Part model, mm, in its own coordinate system. Face numbers are marked on the shaded views. A direction names the side the tool comes from. Coordinates: 2 decimals unless noted, no trailing zeros. Write each loop counter-clockwise with the first axis right and the second up, starting at its lowest first coordinate (ties: lowest second). Pieces come first, ordered by that corner, then holes. Notation, with made-up numbers: (71.5, -33) -> (123.5, -33) arc R29 cw to (123.5, 1) -> close; hole circle Ø5 at (-6, 11.5). An arc over 180 degrees is marked (long way). Write item = value, one per line.
from build123d import *

# Parameters (mm, degrees)
BASE_FLANGE1_DEPTH = 50
EDGE_FLANGE1_DEPTH = 62
SKETCH9_W          = 25
SKETCH9_H          = 20
CUT_EXTRUDE1_DEPTH = 10
EDGE_FLANGE2_DEPTH = 21
SKETCH13_R         = 3.5
CUT_EXTRUDE2_DEPTH = 10
EDGE_FLANGE3_DEPTH = 24
SKETCH17_R         = 6.5
CUT_EXTRUDE3_DEPTH = 10


# Sheet-metal steps are written as plain solids
with BuildPart() as part:
    # Sketch1 → Base-Flange1 (new body)
    with BuildSketch(Plane.YZ):
        with BuildLine():
            Line((-52, 46), (-46, 46))
            ThreePointArc((-46, 46), (-43.171572875, 44.828427125), (-42, 42))
            Line((-42, 42), (-42, 2))
            ThreePointArc((-42, 2), (-41.414213562, 0.585786438), (-40, 0))
            Line((-40, 0), (40, 0))
            ThreePointArc((40, 0), (41.414213562, 0.585786438), (42, 2))
            Line((42, 2), (42, 42))
            ThreePointArc((42, 42), (43.171572875, 44.828427125), (46, 46))
            Line((46, 46), (52, 46))
            Line((52, 46), (52, 44))
            Line((52, 44), (46, 44))
            ThreePointArc((46, 44), (44.585786438, 43.414213562), (44, 42))
            Line((44, 42), (44, 2))
            ThreePointArc((44, 2), (42.828427125, -0.828427125), (40, -2))
            Line((40, -2), (-40, -2))
            ThreePointArc((-40, -2), (-42.828427125, -0.828427125), (-44, 2))
            Line((-44, 2), (-44, 42))
            ThreePointArc((-44, 42), (-44.585786438, 43.414213562), (-46, 44))
            Line((-46, 44), (-52, 44))
            Line((-52, 44), (-52, 46))
        make_face()
    extrude(amount=-BASE_FLANGE1_DEPTH)

    # Edge-Flange1 section (across the edge) → Edge-Flange1 (add)
    with BuildSketch(Plane(origin=(2, -31, 0), x_dir=(-1, 0, 0), z_dir=(0, 1, 0))):
        with BuildLine():
            Line((-2, 2), (-2, 40))
            Line((-2, 40), (0, 40))
            Line((0, 40), (0, 2))
            ThreePointArc((0, 2), (0.585786438, 0.585786438), (2, 0))
            Line((2, 0), (2, -2))
            ThreePointArc((2, -2), (-0.828427125, -0.828427125), (-2, 2))
        make_face()
    extrude(amount=EDGE_FLANGE1_DEPTH)

    # Sketch9 → Cut-Extrude1 (cut)
    with BuildSketch(Plane.YZ.offset(4)):
        with Locations((-14.5, 24)):
            Rectangle(SKETCH9_W, SKETCH9_H)
    extrude(amount=-CUT_EXTRUDE1_DEPTH, mode=Mode.SUBTRACT)

    # Edge-Flange2 section (across the edge) → Edge-Flange2 (add)
    with BuildSketch(Plane(origin=(4, -4, 16), x_dir=(0, 0, -1), z_dir=(0, -1, 0))):
        with BuildLine():
            Line((-2, 2), (-2, 18))
            Line((-2, 18), (0, 18))
            Line((0, 18), (0, 2))
            ThreePointArc((0, 2), (0.585786438, 0.585786438), (2, 0))
            Line((2, 0), (2, -2))
            ThreePointArc((2, -2), (-0.828427125, -0.828427125), (-2, 2))
        make_face()
    extrude(amount=EDGE_FLANGE2_DEPTH)

    # Sketch13 → Cut-Extrude2 (cut)
    with BuildSketch(Plane.XY.offset(18)):
        with Locations((17, -14.5)):
            Circle(SKETCH13_R)
    extrude(amount=-CUT_EXTRUDE2_DEPTH, mode=Mode.SUBTRACT)

    # Edge-Flange3 section (across the edge) → Edge-Flange3 (add)
    with BuildSketch(Plane(origin=(2, 7, 42), x_dir=(0, 0, -1), z_dir=(0, 1, 0))):
        with BuildLine():
            Line((-2, 2), (-2, 33))
            Line((-2, 33), (0, 33))
            Line((0, 33), (0, 2))
            ThreePointArc((0, 2), (0.585786438, 0.585786438), (2, 0))
            Line((2, 0), (2, -2))
            ThreePointArc((2, -2), (-0.828427125, -0.828427125), (-2, 2))
        make_face()
    extrude(amount=EDGE_FLANGE3_DEPTH)

    # Sketch17 → Cut-Extrude3 (cut)
    with BuildSketch(Plane.XY.offset(44)):
        with Locations((-17, 19)):
            Circle(SKETCH17_R)
    extrude(amount=-CUT_EXTRUDE3_DEPTH, mode=Mode.SUBTRACT)


solid = part.part
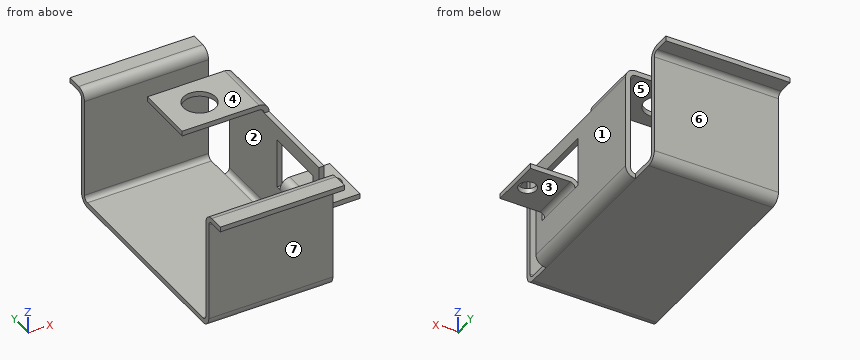
Q1. Pin check, flat tips, straight feed: pin 1 (4 mm diameter, centred on x = -40.5, y = 8, fed in from +Z); pin 2 (10 mm diameter, centred on x = 11.5, y = -15.5, fed in from -Z); pin 3 (21 mm diameter, centred on x = -17, y = 19, fed in from +Z). Stop position of each tip, or through.
Model answer:
pin_1 = 0
pin_2 = 16
pin_3 = 44
Q2. Saw through at A-A on z = 28. Give the cut face in (x, y), and give its area (3 significant figures).
Model answer:
outline = (-50, -44) -> (0, -44) -> (0, -42) -> (-50, -42) -> close; (-50, 42) -> (0, 42) -> (0, 44) -> (-50, 44) -> close; (2, -31) -> (4, -31) -> (4, -27) -> (2, -27) -> close; (2, -2) -> (4, -2) -> (4, 31) -> (2, 31) -> close
area = 274 mm²
Q3. Mould opens along Z. For the marked faces 1, 2 and 3 say: released by +Z, released by -Z, zero draft, split by the parting line, or undercut.
Model answer:
face_1 = zero draft
face_2 = undercut
face_3 = released by -Z
Q4. Saw through at C-C on z = 36.5. Give the cut face in (x, y), and give its area (3 significant figures).
Model answer:
outline = (-50, -44) -> (0, -44) -> (0, -42) -> (-50, -42) -> close; (-50, 42) -> (0, 42) -> (0, 44) -> (-50, 44) -> close; (2, -31) -> (4, -31) -> (4, 31) -> (2, 31) -> close
area = 324 mm²
Q5. Which spindle directions (+Z, -Z, +X, -X, +Y, -Y) get a long thin tool onto all of the face, cutting with end or side? Do the marked faces 4, 5, 6 and 7. Say none if no direction does.
Model answer:
face_4 = +Z, +X, -X
face_5 = -X
face_6 = -Z, +X, -X, +Y
face_7 = -Z, +X, -X, -Y
Q6. Saw through at B-B on y = -14.5. Give the cut face in (x, z), and give its area (3 significant figures).
Model answer:
outline = (-50, -2) -> (0, -2) arc R4 ccw to (4, 2) -> (4, 14) arc R2 cw to (6, 16) -> (13.5, 16) -> (13.5, 18) -> (6, 18) arc R4 ccw to (2, 14) -> (2, 2) arc R2 cw to (0, 0) -> (-50, 0) -> close; (2, 34) -> (4, 34) -> (4, 40) -> (2, 40) -> close; (20.5, 16) -> (22, 16) -> (22, 18) -> (20.5, 18) -> close
area = 173 mm²
Q7. Probe line 1 (Y direction, x = -1.5, z = 2); line 2 (Y direction, x = -17, z = 42.5); line 3 (Z direction, x = -26.5, y = 19). List the from-to ranges inside material, lowest first. Write a range as from..to.
Model answer:
line_1 = -44..-42, 42..44
line_2 = -44.06..-42.03, 7..12.5, 25.5..31, 42.03..44.06
line_3 = -2..0, 42..44
Q8. Saw through at D-D on x = -28.5. Give the cut face in (y, z), and give its area (3 significant figures).
Model answer:
outline = (-52, 44) -> (-46, 44) arc R2 cw to (-44, 42) -> (-44, 2) arc R4 ccw to (-40, -2) -> (40, -2) arc R4 ccw to (44, 2) -> (44, 42) arc R2 cw to (46, 44) -> (52, 44) -> (52, 46) -> (46, 46) arc R4 ccw to (42, 42) -> (42, 2) arc R2 cw to (40, 0) -> (-40, 0) arc R2 cw to (-42, 2) -> (-42, 42) arc R4 ccw to (-46, 46) -> (-52, 46) -> close; (7, 42) -> (31, 42) -> (31, 44) -> (7, 44) -> close
area = 430 mm²
